Could you check a few things on this model? Use its own coordinates, in mm. A direction names the side the tool comes from. Give positions to 0.01 mm unless a question says otherwise; leave off trailing zeros. Order: outer loops, then holes, each group sorted by start corner. A loop starts at its lowest first (then second) coordinate and runs counter-clockwise, first axis right, second up. Notation, with made-up numbers: M 66,74.5 L 76,74.5 A27 cw 76,92.5 Z; hole C -0.5,-39 d3. An arc over 180 degrees is marked long. Use a Markdown table: item, result. Add a question column.
Item 1: If we mould it in two halves opening along X, with no side actions, what happens to faces 6 (the face through (-15.11, 19.525, 68.685)), 7 (the face through (0.716, 11.142, 38.994)), 8 (the face through (54.25, 8.93, 4.93)), 9 (the face through (0, -7, 34.58))? For each: released by +X, released by -X, zero draft, split by the parting line, or undercut.
Item 2: Suppose I cut it at D-D on y = -8. Write out the boundary of the cut face in (x, z).
Item 3: Suppose I cut it at A-A on z = 19. Write out the boundary of the cut face in (x, y), plus the area to 3 significant figures.
Item 4: Suppose I cut it at B-B on x = -51. Write out the boundary of the cut face in (y, z), plus the area to 3 significant figures.
Item 5: Suppose I cut it at C-C on y = 14. Write out the boundary of the cut face in (x, z).
Item 6: If I drill on L1, parallel to Z at x = -44, y = -19.5; L2, parallel to X at y = 2, z = 20; L3, parallel to Y at x = -6.5, z = 41, over which ranges is the centre line in solid material (lowest first)? Write a range as from..to.
Item 7: For faces 1 (the face through (-28, 26.235, 19)), 2 (the face through (-61.839, 0, 5)), 3 (the face through (0, 26.433, 42)), 4 (the face through (0, 6.216, 36)), 5 (the face through (27, 26.235, 19)), which set-ups out of +Z, -Z, +X, -X, +Y, -Y let a thin tool reach every point of the face, with its end or its side?
Item 8: I'm going to push flat-ended pins straight in: pin 1 Ø12 at (y, z) = (-9.5, 34.5) entering from -X; pin 2 Ø13 at (x, y) = (1, -8.5) entering from +Z; pin 3 Ø2 at (x, z) = (2, 36) entering from +Y. Where does each tip first touch, or does it pass through?
from build123d import *

# Parameters (mm, degrees)
SKETCH_R        = 7.84144
PAD_DEPTH       = 10
SKETCH001_W     = 42.19746
SKETCH001_H     = 14.012741
PAD001_DEPTH    = 65
FILLET_R        = 21
SKETCH002_R     = 10.429862
POCKET_DEPTH    = 14.345294
PAD002_DEPTH    = 53
POCKET001_DEPTH = 53.530348
SKETCH005_W     = 26.334992
SKETCH005_H     = 10.429696
POCKET002_DEPTH = 82.9392


with BuildPart() as part:
    # Sketch → Pad (new body)
    with BuildSketch(Plane.XY):
        with BuildLine():
            ThreePointArc((-47.004433, 26.764674), (-57.494388, 22.419592), (-61.83947, 11.929637))
            Line((-61.83947, -11.929637), (-61.83947, 11.929637))
            ThreePointArc((-61.83947, -11.929637), (-57.494388, -22.419592), (-47.004433, -26.764674))
            Line((47.004433, -26.764674), (-47.004433, -26.764674))
            ThreePointArc((47.004433, -26.764674), (57.494388, -22.419592), (61.83947, -11.929637))
            Line((61.83947, 11.929637), (61.83947, -11.929637))
            ThreePointArc((61.83947, 11.929637), (57.494388, 22.419592), (47.004433, 26.764674))
            Line((-47.004433, 26.764674), (47.004433, 26.764674))
        make_face()
        with Locations((-47.004433, 11.929637)):
            Circle(SKETCH_R, mode=Mode.SUBTRACT)
        with Locations((-47.004433, -11.929637)):
            Circle(SKETCH_R, mode=Mode.SUBTRACT)
        with Locations((47.004433, 11.929637)):
            Circle(SKETCH_R, mode=Mode.SUBTRACT)
        with Locations((47.004433, -11.929637)):
            Circle(SKETCH_R, mode=Mode.SUBTRACT)
    extrude(amount=PAD_DEPTH)

    # Sketch001 (on Face14 of Pad) → Pad001 (join)
    with BuildSketch(Plane.XY.offset(10)):
        with Locations((0, 19.426751)):
            Rectangle(SKETCH001_W, SKETCH001_H)
    extrude(amount=PAD001_DEPTH)

    # Fillet
    fillet_edges = [part.edges().sort_by_distance(p)[0] for p in [
        (21.09873, 19.426751, 75),
        (-21.09873, 19.426751, 75),
    ]]
    fillet(fillet_edges, radius=FILLET_R)

    # Sketch002 (on Face5 of Fillet) → Pocket (cut, through all)
    with BuildSketch(Plane.XZ.offset(-12.42038)):
        with Locations((0, 57.346222)):
            Circle(SKETCH002_R)
    extrude(amount=-POCKET_DEPTH, mode=Mode.SUBTRACT)

    # Sketch003 (on Face16 of Pocket) → Pad002 (join)
    with BuildSketch(Plane.XZ.offset(26.764674)):
        with BuildLine():
            ThreePointArc((39.000746, 0), (0, 39.000746), (-39.000746, 0))
            Line((-39.000746, 0), (39.000746, 0))
        make_face()
    extrude(amount=-PAD002_DEPTH)

    # Sketch004 (on Face24 of Pad002) → Pocket001 (cut, through all)
    with BuildSketch(Plane.XZ.offset(26.764674)):
        with BuildLine():
            ThreePointArc((23.640903, -0.107932), (0, 23.641149), (-23.640903, -0.107932))
            Line((-23.640903, -0.107932), (23.640903, -0.107932))
        make_face()
    extrude(amount=-POCKET001_DEPTH, mode=Mode.SUBTRACT)

    # Sketch005 (on DatumPlane) → Pocket002 (cut, through all)
    with BuildSketch(Plane.YZ.offset(21.09873)):
        with Locations((-6.951761, 39.794678)):
            Rectangle(SKETCH005_W, SKETCH005_H)
    extrude(amount=-POCKET002_DEPTH, mode=Mode.SUBTRACT)


solid = part.part
Findings below:
| question | item | result |
|---|---|---|
| 1 | face 6 | released by -X |
| 1 | face 7 | split by the parting line |
| 1 | face 8 | undercut |
| 1 | face 9 | zero draft |
| 2 | outline | M -61.84,0 L -53.79,0 L -53.79,10 L -61.84,10 Z; M -40.22,0 L -23.64,0 A23.64 cw 23.64,0 L 40.22,0 L 40.22,10 L 37.7,10 A39 ccw 18.04,34.58 L -18.04,34.58 A39 ccw -37.7,10 L -40.22,10 Z; M 53.79,0 L 61.84,0 L 61.84,10 L 53.79,10 Z |
| 3 | outline | M -34.06,-26.76 L -14.07,-26.76 L -14.07,26.43 L -21.1,26.43 L -21.1,26.24 L -34.06,26.24 Z; M 14.07,-26.76 L 34.06,-26.76 L 34.06,26.24 L 21.1,26.24 L 21.1,26.43 L 14.07,26.43 Z |
| 3 | area | 2,120 mm^2 |
| 4 | outline | M -26.22,0 L -18.68,0 L -18.68,10 L -26.22,10 Z; M -5.18,0 L 5.18,0 L 5.18,10 L -5.18,10 Z; M 18.68,0 L 26.22,0 L 26.22,10 L 18.68,10 Z |
| 4 | area | 254 mm^2 |
| 5 | outline | M -61.69,0 L -54.57,0 L -54.57,10 L -61.69,10 Z; M -39.44,0 L -23.64,0 A23.64 cw 23.64,0 L 39.44,0 L 39.44,10 L 37.7,10 A39 ccw 21.1,32.8 L 21.1,54 A21 ccw 0.1,75 L -0.1,75 A21 ccw -21.1,54 L -21.1,32.8 A39 ccw -37.7,10 L -39.44,10 Z; M 54.57,0 L 61.69,0 L 61.69,10 L 54.57,10 Z; hole C 0,57.35 d20.86 |
| 6 | L1 | z = 0..10 |
| 6 | L2 | x = -33.48..-12.61, 12.61..33.48 |
| 6 | L3 | y = 12.42..26.43 |
| 7 | face 1 | +Z, -X, +Y |
| 7 | face 2 | +Z, -Z, -X, +Y, -Y |
| 7 | face 3 | +Z, -Z, +X, -X, +Y |
| 7 | face 4 | +Z, +X, -X |
| 7 | face 5 | +Z, +X, +Y |
| 8 | pin 1 | stops at x = -26.62 |
| 8 | pin 2 | stops at z = 34.58 |
| 8 | pin 3 | stops at y = 26.43 |
